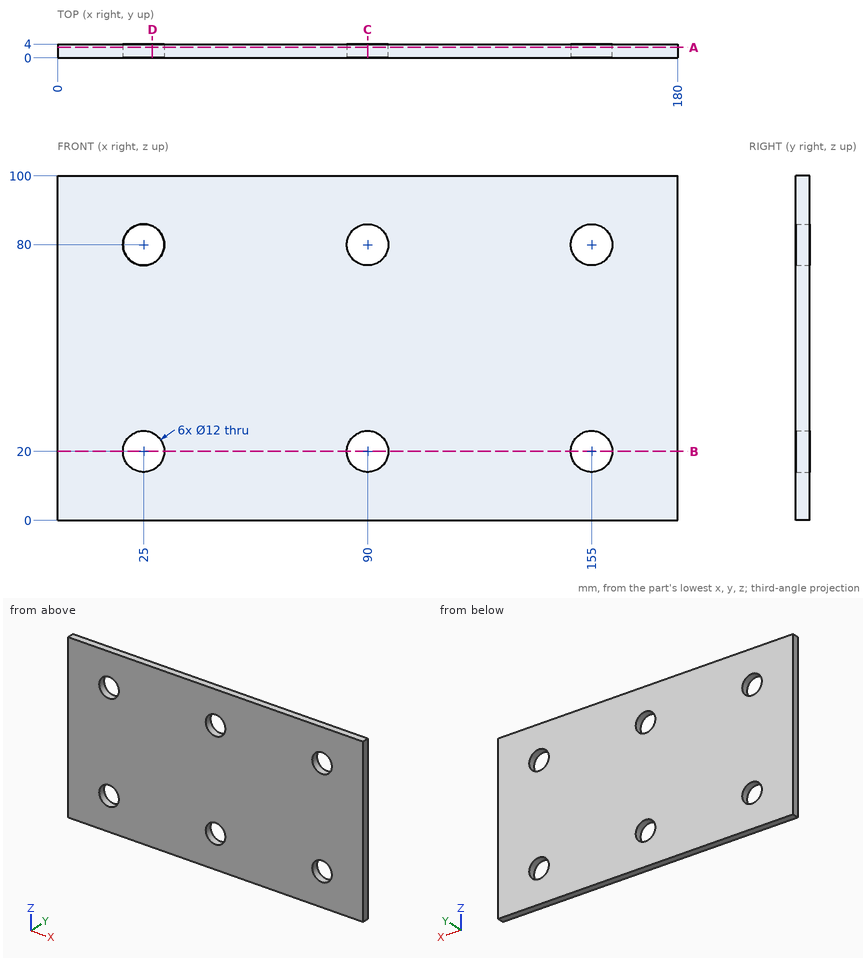
Here's the drawing with two shaded views (mm, measured from the low corner). I have some questions. Round coordinates to 2 decimals unless told otherwise and drop trailing zeros. Order: outer loops, then holes, each group sorted by start corner. A loop starts at its lowest first (then second) coordinate and runs counter-clockwise, first axis right, second up. Notation, with made-up numbers: (68, 26) -> (126, 26) arc R30 cw to (126, 54) -> close; hole circle Ø10 at (-28.5, 51). An arc over 180 degrees is marked (long way). Write each question's results on one line, items separated by ' | '. Start each with the question number.
Item 1: If we section it at A-A, the plane y = 3: Write out the boundary of the cut face in (x, z), then the cut area to 3 significant figures.
Item 2: If we section it at B-B, the plane z = 20: Write out the boundary of the cut face in (x, y).
Item 3: If we section it at C-C, the plane x = 90: Write out the boundary of the cut face in (y, z).
Item 4: If we section it at D-D, the plane x = 27.5: Write out the boundary of the cut face in (y, z).
Item 5: Will these pins go through, and if not, where does the flat tip stop? pin 1 (19 mm diameter, centred on x = 155, z = 80, fed in from +Y); pin 2 (9.5 mm diameter, centred on x = 155, z = 20, fed in from +Y).
Item 6: Please list where these lines run through material, in increasing order: L1, parallel to Z at x = 90, y = 3.1; L2, parallel to Z at x = 20, y = 0.45; L3, parallel to X at y = 1.5, z = 24.5.
Results:
1) outline: (0, 0) -> (180, 0) -> (180, 100) -> (0, 100) -> close; hole circle Ø12 at (25, 20); hole circle Ø12 at (25, 80); hole circle Ø12 at (90, 20); hole circle Ø12 at (90, 80); hole circle Ø12 at (155, 20); hole circle Ø12 at (155, 80) | area: 17,300 mm2
2) outline: (0, 0) -> (19, 0) -> (19, 4) -> (0, 4) -> close; (31, 0) -> (84, 0) -> (84, 4) -> (31, 4) -> close; (96, 0) -> (149, 0) -> (149, 4) -> (96, 4) -> close; (161, 0) -> (180, 0) -> (180, 4) -> (161, 4) -> close
3) outline: (0, 0) -> (4, 0) -> (4, 14) -> (0, 14) -> close; (0, 26) -> (4, 26) -> (4, 74) -> (0, 74) -> close; (0, 86) -> (4, 86) -> (4, 100) -> (0, 100) -> close
4) outline: (0, 0) -> (4, 0) -> (4, 14.55) -> (0, 14.55) -> close; (0, 25.45) -> (4, 25.45) -> (4, 74.55) -> (0, 74.55) -> close; (0, 85.45) -> (4, 85.45) -> (4, 100) -> (0, 100) -> close
5) pin 1: stops at y = 4 | pin 2: passes through
6) L1: z = 0 to 14, 26 to 74, 86 to 100 | L2: z = 0 to 16.68, 23.32 to 76.68, 83.32 to 100 | L3: x = 0 to 21.03, 28.97 to 86.03, 93.97 to 151.03, 158.97 to 180
